Build history of the part. All positions in model axes, mm. A direction names the side the tool comes from. Give positions to 0.01 mm unless a question says otherwise; leave off trailing zeros. Order: outer loops, then holes, each group sorted by start corner. A loop starts at its lowest first (then second) coordinate and runs counter-clockwise, first axis right, second up. Notation, with made-up numbers: (5, 29.5) -> (20, 29.5) arc R32 cw to (20, 63.5) -> close; hole circle Ø7 at (52.25, -33.5). An arc over 180 degrees is marked (long way). One line per item, written item: value. Start each with the question number.
(1) Two-plate mould, pull along Y, no slides. Class faces 1 (the flat face through (-47, 6, 10.16)), 2 (the flat face through (-4, 15.24, 33)), 3 (the cylindrical face through (41.105, 1.288, -26.644)): +Y half, -Y half, draft (parallel to the pull), parting line (faces both ways), or undercut.
(2) Saw through at D-D on x = 39.37. Give the cut face in (y, z).
(3) Saw through at C-C on y = 13.5. Give the cut face in (x, z).
(4) Pin check, flat tips, straight feed: pin 1 (2 mm diameter, centred on x = 39.37, z = 25.654, fed in from -Y); pin 2 (4 mm diameter, centred on x = 39.37, z = -26.416, fed in from +Y). Stop position of each tip, or through.
(5) Which spindle directions (+Z, -Z, +X, -X, +Y, -Y) get a long thin tool onto all of the face, cutting with end or side? Do faces 4 (the flat face through (-45.72, 10, 0)), 5 (the cylindrical face through (41.1, 1.3, 25.4)), 6 (the flat face through (-47, 6, -3.81)). Say none if no direction does.
(6) Saw through at A-A on x = -40.64. Give the cut face in (y, z), plus the area to 3 significant figures.
(7) Probe line 1 (X direction, y = 1.7, z = -26.67); line 2 (Z direction, x = -0.5, y = 3.75); line 3 (X direction, y = 3, z = 16.5). List the from-to ranges inside material, lowest first.
(8) Saw through at B-B on z = 6.5. Give the cut face in (x, y).
```python
from build123d import *

# Parameters (mm, degrees)
SKETCH1_W           = 96.52
SKETCH1_H           = 68.58
BOSS_EXTRUDE2_DEPTH = 2.54
SKETCH4_W           = 96.52
SKETCH4_H           = 68.58
SKETCH4_W_2         = 91.44
SKETCH4_H_2         = 63.5
BOSS_EXTRUDE3_DEPTH = 12.7
SKETCH5_W           = 13.97
SKETCH5_H           = 6.35
CUT_EXTRUDE2_DEPTH  = 12.7
SKETCH6_R           = 1.75
CUT_EXTRUDE4_DEPTH  = 2.54


with BuildPart() as part:
    # Sketch1 → Boss-Extrude2 (new body)
    with BuildSketch(Plane(origin=(0, 0, 0), x_dir=(1, 0, 0), z_dir=(0, 1, 0))):
        Rectangle(SKETCH1_W, SKETCH1_H)
    extrude(amount=BOSS_EXTRUDE2_DEPTH)

    # Sketch4 → Boss-Extrude3 (add)
    with BuildSketch(Plane(origin=(0, 2.54, 0), x_dir=(1, 0, 0), z_dir=(0, 1, 0))):
        Rectangle(SKETCH4_W, SKETCH4_H)
        Rectangle(SKETCH4_W_2, SKETCH4_H_2, mode=Mode.SUBTRACT)
    extrude(amount=BOSS_EXTRUDE3_DEPTH)

    # Sketch5 → Cut-Extrude2 (cut)
    with BuildSketch(Plane.ZY.offset(48.26)):
        with Locations((3.175, 5.715)):
            Rectangle(SKETCH5_W, SKETCH5_H)
    extrude(amount=-CUT_EXTRUDE2_DEPTH, mode=Mode.SUBTRACT)

    # Sketch6 → Cut-Extrude4 (cut)
    with BuildSketch(Plane(origin=(0, 2.54, 0), x_dir=(1, 0, 0), z_dir=(0, 1, 0))):
        with Locations(Location((-40.64, 26.67, 0), (0, 0, 270))):
            Circle(SKETCH6_R)
        with Locations(Location((39.37, 26.416, 0), (0, 0, 270))):
            Circle(SKETCH6_R)
        with Locations(Location((39.37, -25.654, 0), (0, 0, 270))):
            Circle(SKETCH6_R)
    extrude(amount=-CUT_EXTRUDE4_DEPTH, mode=Mode.SUBTRACT)


solid = part.part
```
Results below:
1. face 1: undercut
1. face 2: +Y half
1. face 3: draft
2. outline: (0, -34.29) -> (15.24, -34.29) -> (15.24, -31.75) -> (2.54, -31.75) -> (2.54, -28.17) -> (0, -28.17) -> close; (0, -24.67) -> (2.54, -24.67) -> (2.54, 23.9) -> (0, 23.9) -> close; (0, 27.4) -> (2.54, 27.4) -> (2.54, 31.75) -> (15.24, 31.75) -> (15.24, 34.29) -> (0, 34.29) -> close
3. outline: (-48.26, -34.29) -> (48.26, -34.29) -> (48.26, 34.29) -> (-48.26, 34.29) -> close; hole (-45.72, -31.75) -> (45.72, -31.75) -> (45.72, 31.75) -> (-45.72, 31.75) -> close
4. pin 1: passes through
4. pin 2: stops at y = 2.54
5. face 4: +Y
5. face 5: +Y, -Y
5. face 6: -X
6. outline: (0, -34.29) -> (15.24, -34.29) -> (15.24, -31.75) -> (2.54, -31.75) -> (2.54, -28.42) -> (0, -28.42) -> close; (0, -24.92) -> (2.54, -24.92) -> (2.54, 31.75) -> (15.24, 31.75) -> (15.24, 34.29) -> (0, 34.29) -> close
6. area: 230 mm²
7. line 1: x = -48.26 to -42.39, -38.89 to 37.64, 41.1 to 48.26
7. line 2: z = -34.29 to -31.75, 31.75 to 34.29
7. line 3: x = -48.26 to -45.72, 45.72 to 48.26
8. outline: (-48.26, 0) -> (48.26, 0) -> (48.26, 15.24) -> (45.72, 15.24) -> (45.72, 2.54) -> (-48.26, 2.54) -> close; (-48.26, 8.89) -> (-45.72, 8.89) -> (-45.72, 15.24) -> (-48.26, 15.24) -> close
